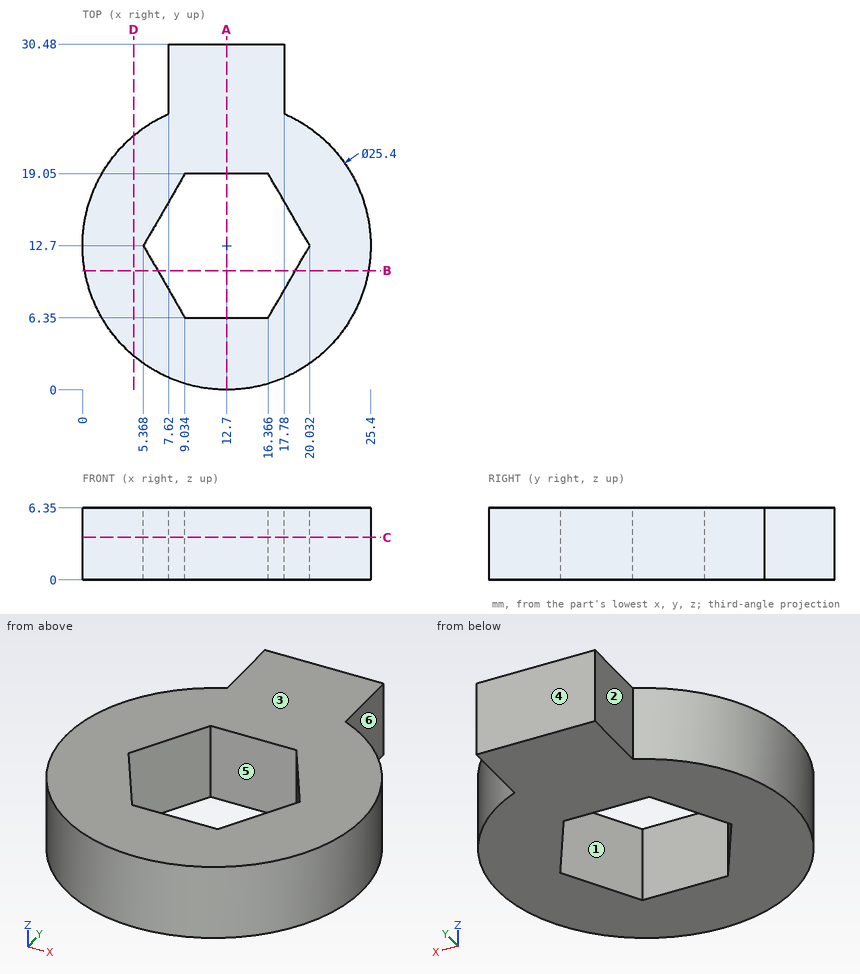
Check sheet for the drawn part. Datum: minimum x, y, z corner. Units: mm. A direction names the side the tool comes from. Give positions to 0.01 mm unless a question says otherwise; leave off trailing zeros. Order: outer loops, then holes, each group sorted by start corner. A loop starts at its lowest first (then second) coordinate and runs counter-clockwise, first axis right, second up.
1. Sectioned sample at C-C (z = 3.75). Record the boundary of the cut face in (x, y), then the cut area to 3 significant figures.
Completed:
outline: (7.62, 24.34) arc R12.7 ccw (long way) to (17.78, 24.34) - (17.78, 30.48) - (7.62, 30.48) - close; hole (5.37, 12.7) - (9.03, 6.35) - (16.37, 6.35) - (20.03, 12.7) - (16.37, 19.05) - (9.03, 19.05) - close
area: 422 mm2
2. Access from +Z, -Z, +X, -X, +Y, -Y to the whole of each face (thin tool, end or side, straight path). Record for the marked faces 1, 2 and 3.
Completed:
face 1: +Z, -Z
face 2: +Z, -Z, -X, +Y
face 3: +Z, +X, -X, +Y, -Y
3. Depth check by flat-ended pin: pin 1 (1.8 mm diameter, centred on y = 26.5, z = 2, fed in from -X); pin 2 (1 mm diameter, centred on x = 21.5, z = 1.5, fed in from -Y); pin 3 (3 mm diameter, centred on y = 20, z = 4.5, fed in from +X); pin 4 (3 mm diameter, centred on x = 3.5, y = 26, fed in from +Z). Enter the tip coordinate at first touch or a pass-through.
Completed:
pin 1: stops at x = 7.62
pin 2: stops at y = 3.09
pin 3: stops at x = 24
pin 4: passes through
4. Draft check along Y on the marked faces 4, 5 and 6. Enter one of: pulls with the +Y half, pulls with the -Y half, needs draft (parallel to the pull), parting line crosses it, or undercut.
Completed:
face 4: pulls with the +Y half
face 5: undercut
face 6: needs draft
5. Sectioned sample at B-B (y = 10.5). Record the boundary of the cut face in (x, z).
Completed:
outline: (0.19, 0) - (6.64, 0) - (6.64, 6.35) - (0.19, 6.35) - close; (18.76, 0) - (25.21, 0) - (25.21, 6.35) - (18.76, 6.35) - close
6. Scan lines: line 1 (Y direction, x = 13, z = 1); line 2 (Y direction, x = 14.75, z = 4.5); line 3 (X direction, y = 8.5, z = 4) (1 decimal). Record each from-to range of solid material in increasing order.
Completed:
line 1: y = 0 to 6.35, 19.05 to 30.48
line 2: y = 0.17 to 6.35, 19.05 to 30.48
line 3: x = 0.7 to 7.8, 17.6 to 24.7
7. Sectioned sample at D-D (x = 4.5). Record the boundary of the cut face in (y, z), then the cut area to 3 significant figures.
Completed:
outline: (3, 0) - (22.4, 0) - (22.4, 6.35) - (3, 6.35) - close
area: 123 mm2
8. Sectioned sample at A-A (x = 12.7). Record the boundary of the cut face in (y, z), then the cut area to 3 significant figures.
Completed:
outline: (0, 0) - (6.35, 0) - (6.35, 6.35) - (0, 6.35) - close; (19.05, 0) - (30.48, 0) - (30.48, 6.35) - (19.05, 6.35) - close
area: 113 mm2
